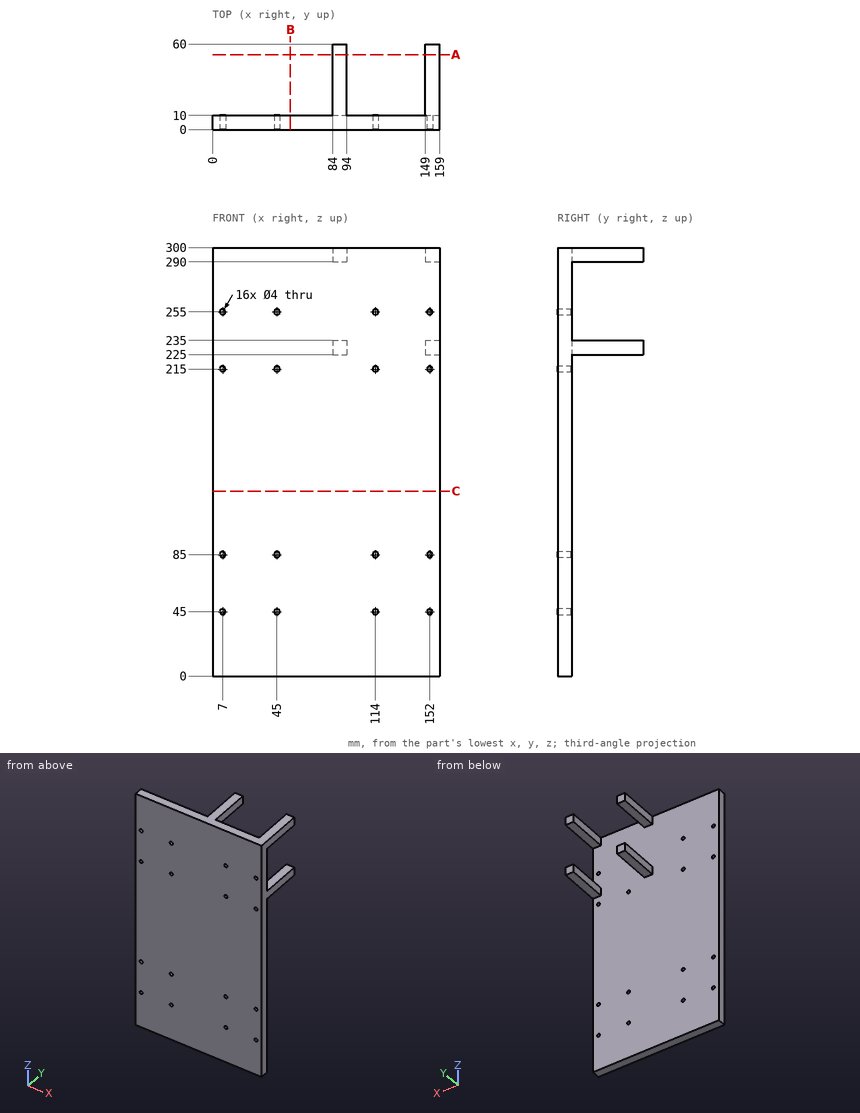
Could you check a few things on this drawing? It's one solid part, dimensions in mm from its lowest x, y, z. Give positions to 0.01 mm unless a question says otherwise; leave off trailing zeros. Order: outer loops, then holes, each group sorted by start corner. A loop starts at its lowest first (then second) coordinate and runs counter-clockwise, first axis right, second up. Notation, with made-up numbers: (-31.5, 8.5) - (-11.5, 8.5) arc R20 cw to (-11.5, 16.5) - close; hole circle Ø11 at (-16, 18.25). An arc over 180 degrees is marked (long way). Answer as a JSON object with one key per item and string values. Group by question number.
Item 1: If we section it at A-A on y = 52.5: Please give me the cut outline in (x, z).
Item 2: If we section it at B-B on x = 54.5: Please give me the cut outline in (y, z).
Item 3: For P1, Ø3, axis at x = 114, z = 45, coming from the -Y side; P2, Ø4, axis at x = 32, z = 138.5, coming from the -Y side; P3, Ø2, axis at x = 118.5, z = 186.5, coming from the +Y side; P4, Ø5, axis at x = 155, y = 35, coming from the -Z side, each with a flat end and sliding along its axis, tell me the tip position at first contact or that it passes through.
Item 4: Please list where these lines run through material, in increasing order: probe 1 along X at (y, z) = (4, 45); probe 2 along Z at (x, y) = (152, 7); probe 3 along Y at (x, z) = (132, 167.5).
Item 5: If we section it at C-C on z = 129.5: Please give me the cut outline in (x, y), and give its area (3 significant figures).
Result set:
{
 "1": {"outline": "(84, 225) - (94, 225) - (94, 235) - (84, 235) - close; (84, 290) - (94, 290) - (94, 300) - (84, 300) - close; (149, 225) - (159, 225) - (159, 235) - (149, 235) - close; (149, 290) - (159, 290) - (159, 300) - (149, 300) - close"},
 "2": {"outline": "(0, 0) - (10, 0) - (10, 300) - (0, 300) - close"},
 "3": {"P1": "through", "P2": "y = 0", "P3": "y = 10", "P4": "z = 225"},
 "4": {"probe 1": "0 to 5, 9 to 43, 47 to 112, 116 to 150, 154 to 159", "probe 2": "0 to 43, 47 to 83, 87 to 213, 217 to 253, 257 to 300", "probe 3": "0 to 10"},
 "5": {"outline": "(0, 0) - (159, 0) - (159, 10) - (0, 10) - close", "area": "1,590 mm²"}
}
